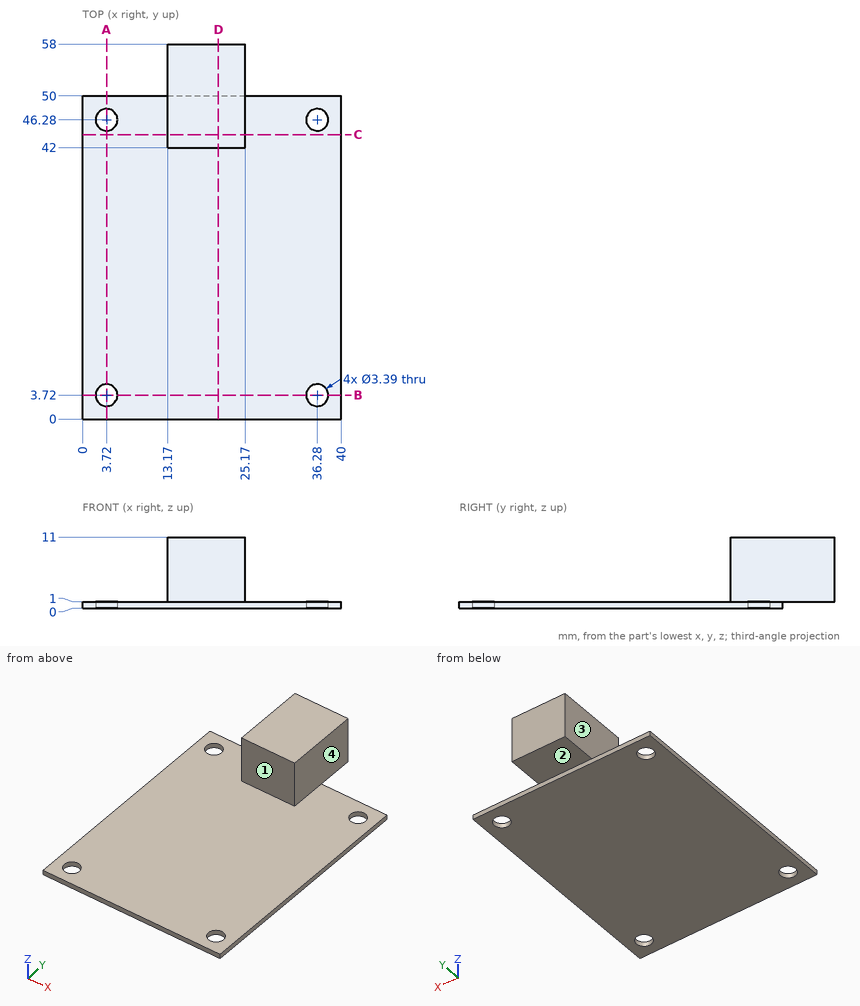
Check sheet for the drawn part. Datum: minimum x, y, z corner. Units: mm. A direction names the side the tool comes from. Round coordinates to 2 decimals unless told otherwise and drop trailing zeros. Order: outer loops, then holes, each group sorted by start corner. A loop starts at its lowest first (then second) coordinate and runs counter-clockwise, first axis right, second up. Notation, with made-up numbers: M 84.25,24.25 L 108.25,24.25 A19 cw 108.25,60.25 Z; hole C -14.75,26 d7. An arc over 180 degrees is marked long. Write each question's results on one line, items separated by ' | '. Start each with the question number.
1. Go/stop test with flat-tipped pins: P1, Ø9, axis at x = 21.5, y = 55.5, coming from the -Z side; P2, Ø1, axis at x = 5.5, y = 32.5, coming from the -Z side; P3, Ø20, axis at x = 19.5, y = 26.5, coming from the +Z side; P4, Ø4, axis at x = 9.5, z = 1.5, coming from the +Y side. Record where each tip stops, or that it passes through.
2. Cross-section at B-B on y = 3.72. Record the boundary of the cut face in (x, z) (3 decimals).
3. Set-up check for the marked faces 1, 2, 3 and 4: record each of +Z, -Z, +X, -X, +Y, -Y from which the full face is reachable in a straight line by a thin tool's end or side.
4. Cross-section at C-C on y = 44. Record the boundary of the cut face in (x, z).
5. Cross-section at A-A on x = 3.72. Record the boundary of the cut face in (y, z) (3 decimals).
6. Material ranges on L1, parallel to Y at x = 36.28, z = 0.55 (3 decimals); L2, parallel to Z at x = 25, y = 30.5; L3, parallel to Y at x = 17, z = 9.5, recorded low to high. Write a range as from..to.
7. Cross-section at D-D on x = 21. Record the boundary of the cut face in (y, z).
Resolved:
1) P1: z = 1 | P2: z = 0 | P3: z = 1 | P4: y = 50
2) outline: M 0,0 L 2.025,0 L 2.025,1 L 0,1 Z; M 5.415,0 L 34.585,0 L 34.585,1 L 5.415,1 Z; M 37.975,0 L 40,0 L 40,1 L 37.975,1 Z
3) face 1: +Z, +X, -X, -Y | face 2: -Z, +X, -X, +Y | face 3: +Z, -X, +Y, -Y | face 4: +Z, +X, +Y, -Y
4) outline: M 0,0 L 40,0 L 40,1 L 25.17,1 L 25.17,11 L 13.17,11 L 13.17,1 L 0,1 Z
5) outline: M 0,0 L 2.025,0 L 2.025,1 L 0,1 Z; M 5.415,0 L 44.585,0 L 44.585,1 L 5.415,1 Z; M 47.975,0 L 50,0 L 50,1 L 47.975,1 Z
6) L1: 0..2.025, 5.415..44.585, 47.975..50 | L2: 0..1 | L3: 42..58
7) outline: M 0,0 L 50,0 L 50,1 L 58,1 L 58,11 L 42,11 L 42,1 L 0,1 Z
